from build123d import *

# Parameters (mm, degrees)
SKETCH1_W           = 23.5
SKETCH1_H           = 23
BOSS_EXTRUDE1_DEPTH = 1.65
SKETCH2_W           = 4.4
SKETCH2_H           = 5
BOSS_EXTRUDE2_DEPTH = 1.55
CUT_EXTRUDE1_REACH  = 34.924
SKETCH3_W           = 3
SKETCH3_H           = 10.5
CUT_EXTRUDE2_REACH  = 34.924
SKETCH4_W           = 3
SKETCH4_H           = 8
CUT_EXTRUDE3_REACH  = 34.924
SKETCH5_R           = 1.8
SKETCH5_R_2         = 1.95


with BuildPart() as part:
    # Sketch1 → Boss-Extrude1 (new body)
    with BuildSketch(Plane.XY):
        with Locations((11.75, 11.5)):
            Rectangle(SKETCH1_W, SKETCH1_H)
    extrude(amount=BOSS_EXTRUDE1_DEPTH)

    # Sketch2 → Boss-Extrude2 (add)
    with BuildSketch(Plane.XY.offset(1.65)):
        with Locations((11.6, 11.5)):
            Rectangle(SKETCH2_W, SKETCH2_H)
    extrude(amount=BOSS_EXTRUDE2_DEPTH)

    # Sketch3 → Cut-Extrude1 (cut, up to next)
    with BuildSketch(Plane.XY.offset(1.65), mode=Mode.PRIVATE) as cut_extrude1_sk1:
        with Locations((18, 12.25)):
            Rectangle(SKETCH3_W, SKETCH3_H)
    cut_extrude1_tool1 = extrude(cut_extrude1_sk1.sketch, amount=-CUT_EXTRUDE1_REACH, mode=Mode.PRIVATE) & part.part
    add(cut_extrude1_tool1.solids().sort_by_distance((18, 12.25, 1.65))[0], mode=Mode.SUBTRACT)

    # Sketch4 → Cut-Extrude2 (cut, up to next)
    with BuildSketch(Plane.XY.offset(1.65), mode=Mode.PRIVATE) as cut_extrude2_sk1:
        with Locations((4.8, 11.3)):
            Rectangle(SKETCH4_W, SKETCH4_H)
    cut_extrude2_tool1 = extrude(cut_extrude2_sk1.sketch, amount=-CUT_EXTRUDE2_REACH, mode=Mode.PRIVATE) & part.part
    add(cut_extrude2_tool1.solids().sort_by_distance((4.8, 11.3, 1.65))[0], mode=Mode.SUBTRACT)

    # Sketch5 → Cut-Extrude3 (cut, up to next)
    with BuildSketch(Plane.XY.offset(1.65), mode=Mode.PRIVATE) as cut_extrude3_sk1:
        with Locations((3.7, 19.25)):
            Circle(SKETCH5_R)
    cut_extrude3_tool1 = extrude(cut_extrude3_sk1.sketch, amount=-CUT_EXTRUDE3_REACH, mode=Mode.PRIVATE) & part.part
    # Sketch5 → Cut-Extrude3 (cut, up to next)
    with BuildSketch(Plane.XY.offset(1.65), mode=Mode.PRIVATE) as cut_extrude3_sk2:
        with Locations((19.95, 19.5)):
            Circle(SKETCH5_R_2)
    cut_extrude3_tool2 = extrude(cut_extrude3_sk2.sketch, amount=-CUT_EXTRUDE3_REACH, mode=Mode.PRIVATE) & part.part
    # Sketch5 → Cut-Extrude3 (cut, up to next)
    with BuildSketch(Plane.XY.offset(1.65), mode=Mode.PRIVATE) as cut_extrude3_sk3:
        with Locations((19.7, 3.7)):
            Circle(SKETCH5_R)
    cut_extrude3_tool3 = extrude(cut_extrude3_sk3.sketch, amount=-CUT_EXTRUDE3_REACH, mode=Mode.PRIVATE) & part.part
    # Sketch5 → Cut-Extrude3 (cut, up to next)
    with BuildSketch(Plane.XY.offset(1.65), mode=Mode.PRIVATE) as cut_extrude3_sk4:
        with Locations((3.66, 3.5)):
            Circle(SKETCH5_R)
    cut_extrude3_tool4 = extrude(cut_extrude3_sk4.sketch, amount=-CUT_EXTRUDE3_REACH, mode=Mode.PRIVATE) & part.part
    add(cut_extrude3_tool1.solids().sort_by_distance((3.7, 19.25, 1.65))[0], mode=Mode.SUBTRACT)
    add(cut_extrude3_tool2.solids().sort_by_distance((19.95, 19.5, 1.65))[0], mode=Mode.SUBTRACT)
    add(cut_extrude3_tool3.solids().sort_by_distance((19.7, 3.7, 1.65))[0], mode=Mode.SUBTRACT)
    add(cut_extrude3_tool4.solids().sort_by_distance((3.66, 3.5, 1.65))[0], mode=Mode.SUBTRACT)


solid = part.part
Verification items for the finished model (mm, model axes). A direction names the side the tool comes from. Give positions to 0.01 mm unless a question says otherwise; leave off trailing zeros. Write each loop counter-clockwise with the first axis right and the second up, starting at its lowest first coordinate (ties: lowest second). Pieces come first, ordered by that corner, then holes. Notation, with made-up numbers: M -37,67 L 11,67 A14 cw 11,82 Z; hole C -20.75,76.5 d11. An arc over 180 degrees is marked long. Put each result on its own line as item: value. Start each with the question number.
1. Section check A-A (x = 21). Record the cut outline in (y, z).
2. Scan lines: line 1 along X through (y, z) = (12.75, 1.6); line 2 along Y through (x, z) = (3.7, 0.75); line 3 along X through (y, z) = (20.25, 0.3). Record each from-to range of solid material in increasing order. Write a range as [from, to].
3. Go/stop test with flat-tipped pins: pin 1 Ø2 at (x, y) = (10, 7.5) entering from +Z; pin 2 Ø0.8 at (x, z) = (11, 2.5) entering from -Y. Record where each tip stops, or that it passes through.
4. Section check B-B (y = 18.25). Record the cut outline in (x, z).
5. Section check C-C (z = 0.4). Record the cut outline in (x, y), and give its area (3 significant figures).
6. Draft check along X on faces 4 (the face through (12, 14, 2)), 5 (the face through (23.5, 11, 1)), 6 (the face through (19.5, 12, 1)). Enter one of: +X half, -X half, draft (parallel to the pull), parting line (faces both ways), or undercut.
7. Section check D-D (x = 18.5). Record the cut outline in (y, z).
8. Set-up check for faces 1 (the face through (9.4, 11, 2)), 2 (the face through (12, 9, 2)), 3 (the face through (5, 7.3, 1)): record each of +Z, -Z, +X, -X, +Y, -Y from which the full face is reachable in a straight line by a thin tool's end or side.
Answer list:
1. outline: M 0,0 L 2.46,0 L 2.46,1.65 L 0,1.65 Z; M 4.94,0 L 17.86,0 L 17.86,1.65 L 4.94,1.65 Z; M 21.14,0 L 23,0 L 23,1.65 L 21.14,1.65 Z
2. line 1: [0, 3.3], [6.3, 16.5], [19.5, 23.5]
2. line 2: [0, 1.7], [5.3, 7.3], [15.3, 17.45], [21.05, 23]
2. line 3: [0, 2.2], [5.2, 18.15], [21.75, 23.5]
3. pin 1: z = 1.65
3. pin 2: y = 9
4. outline: M 0,0 L 2.2,0 L 2.2,1.65 L 0,1.65 Z; M 5.2,0 L 18.45,0 L 18.45,1.65 L 5.2,1.65 Z; M 21.45,0 L 23.5,0 L 23.5,1.65 L 21.45,1.65 Z
5. outline: M 0,0 L 23.5,0 L 23.5,23 L 0,23 Z; hole C 3.66,3.5 d3.6; hole C 3.7,19.25 d3.6; hole M 3.3,7.3 L 6.3,7.3 L 6.3,15.3 L 3.3,15.3 Z; hole M 16.5,7 L 19.5,7 L 19.5,17.5 L 16.5,17.5 Z; hole C 19.7,3.7 d3.6; hole C 19.95,19.5 d3.9
5. area: 443 mm2
6. face 4: draft
6. face 5: +X half
6. face 6: undercut
7. outline: M 0,0 L 2.36,0 L 2.36,1.65 L 0,1.65 Z; M 5.04,0 L 7,0 L 7,1.65 L 5.04,1.65 Z; M 17.5,0 L 18.2,0 L 18.2,1.65 L 17.5,1.65 Z; M 20.8,0 L 23,0 L 23,1.65 L 20.8,1.65 Z
8. face 1: +Z, -X, +Y, -Y
8. face 2: +Z, +X, -X, -Y
8. face 3: +Z, -Z
